Geometry check sheet. Reference: the model listing, model coordinates, mm. Face numbers are marked on the shaded views. A direction names the side the tool comes from. Round coordinates to 2 decimals unless told otherwise and drop trailing zeros. Loops run counter-clockwise (first coordinate to the right, second up) from the corner with the lowest first, then second, coordinate; pieces in that order, holes last. Notation, with made-up numbers: (37, 13.5) -> (43, 13.5) arc R32 ccw to (43, 50.5) -> close; hole circle Ø5 at (-2.75, -28). An arc over 180 degrees is marked (long way). Use a Markdown table: item, result. Add a question column.
Q1. Sectioned sample at A-A, the plane x = 8.75. Enter the section's corners in (y, z) (3 decimals).
Q2. Set-up check for the marked faces 1, 2, 3 and 4: record each of +Z, -Z, +X, -X, +Y, -Y from which the full face is reachable in a straight line by a thin tool's end or side.
Q3. Gauge pin test, flat ends, axial feed: P1, Ø2, axis at x = 1.5, z = 2.5, coming from the +Y side; P2, Ø5, axis at x = -5, y = 1, coming from the -Z side; P3, Ø4, axis at x = 4, z = -4.5, coming from the -Y side; P4, Ø3.5, axis at y = 1.5, z = -2, coming from the +X side (3 decimals). Record the tip position at first contact, or that the pin passes through.
Q4. Material ranges on L1, parallel to X at y = 4.25, z = 2; L2, parallel to X at y = 0, z = 5.5; L3, parallel to Z at x = -1, y = -3.75, recorded low to high.
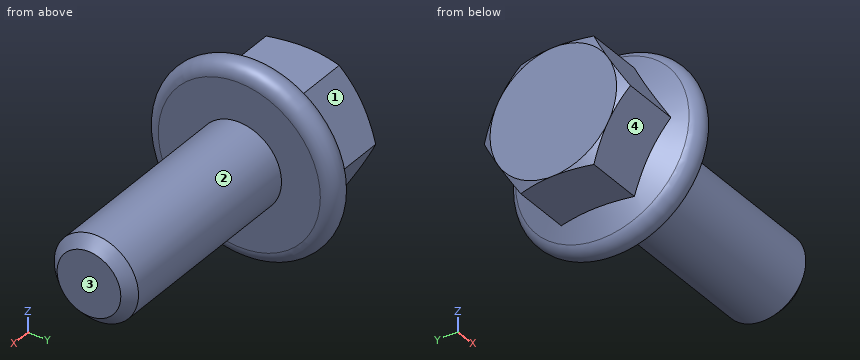
Autodesk Inventor part; units mm, degrees
ref_plane "Work Plane1" through (10.95, 0, 0) normal (0, 0, -1) x (1, 0, 0)
ref_plane "YZ Plane" through (0, 0, 0) normal (1, 0, 0) x (0, 1, 0)
ref_plane "XZ Plane" through (0, 0, 0) normal (0, 1, 0) x (-1, 0, 0)
sketch "Sketch1" plane through (0, 0, 0) normal (0, 0, 1) x (1, 0, 0)
  line L0 (-3.2004, 0) -> (-3.2004, 3.8156)
  line L1 (0, 6.096) -> (0, 3.175)
  line L2 (4.1148, 3.175) -> (15.875, 3.175)
  line L3 (15.875, 3.175) -> (15.875, 0)
  line L4 (15.875, 0) -> (-3.2004, 0)
  arc A0 (0, 6.096) -> (-1.9368, 6.5254) centre (-1.016, 6.096) ccw
  line L5 (0, -1.4605) -> (0, 8.7631)
  line L6 (-7.0155, 0) -> (19.6901, 0)
  line L7 (0, 3.175) -> (0.0001, 3.175)
  line L8 (0.0001, 3.175) -> (0.0001, 3.175)
  line L9 (0.0001, 3.175) -> (2.2098, 3.175)
  line L10 (2.2098, 3.175) -> (4.1148, 3.175)
  line L11 (-3.2004, 3.8156) -> (-1.9368, 6.5254)
  line L12 (0.0001, 3.175) -> (4.1148, 3.175) construction
  line L13 (4.1148, 3.175) -> (4.1148, 0) construction
  dimension "d0" = 1.016
  dimension "d1" = 15.875
  dimension "d2" = 11.7602
  dimension "d3" = 14.224
  dimension "d4" = 6.35
  dimension "d5" = 3.2004
  dimension "d15" = 6.35
  dimension "d16" = 6.35
  dimension "d17" = 0.0001
  dimension "d18" = 1.905
  dimension "d19" = 25
revolve "Body" add sketch "Sketch1" angle 360 about axis through (15.875, 0, 0) along (-1, 0, 0)
sketch "Sketch2" plane through (0, 0, 0) normal (1, 0, 0) x (0, 0, -1)
  line L0 (4.7625, 2.7496) -> (4.7625, -2.7496)
  line L1 (4.7625, -2.7496) -> (0, -5.4993)
  line L2 (0, -5.4993) -> (-4.7625, -2.7496)
  line L3 (-4.7625, -2.7496) -> (-4.7625, 2.7496)
  line L4 (-4.7625, 2.7496) -> (0, 5.4993)
  line L5 (0, 5.4993) -> (4.7625, 2.7496)
  point P0 (0, 0)
  point P1 (0, 0)
  dimension "d23" = 9.525
extrude "Head" add sketch "Sketch2" against normal blind 7.112
sketch "Sketch3" plane through (0, 0, 0) normal (0, 0, 1) x (1, 0, 0)
  line L0 (-7.112, 4.7625) -> (-7.112, 5.4993)
  line L1 (-7.112, 5.4993) -> (-6.6866, 5.4993)
  line L2 (-6.6866, 5.4993) -> (-7.112, 4.7625)
  line L3 (-8.0513, 0) -> (-1.476, 0)
  line L4 (-7.112, 5.4993) -> (-7.112, 2.7496)
  line L5 (-2.4153, 5.4993) -> (-7.112, 5.4993)
  point P0 (-7.112, 2.7496)
  dimension "d8" = 30
  dimension "d22" = 9.525
revolve "Chamfer1" cut sketch "Sketch3" angle 360 about axis through (-10, 0, 0) along (1, 0, 0)
thread "Thread"
chamfer "Chamfer2" distance 0.7791 distance2 0.7791 1 edges at (15.875, -3.175, 0) measured on face at (15.875, 0.0371, -1.7957)
ref_plane "Work Plane1" through (10.95, 0, 0) normal (0, 0, -1) x (1, 0, 0)
equation "\"d23\" = SW"
equation "\"d6\" = KOH"
equation "\"d10\" = GEL"
equation "\"d13\" = -0.5 * SPD + 0.5 * GD"
equation "\"d14\" = GUL"
equation "\"d0\" = PHH"
equation "\"d1\" = NLG"
equation "\"d2\" = GEL"
equation "\"d3\" = LADI"
equation "\"d4\" = GD"
equation "\"d5\" = 0.45 * KOH"
equation "\"d15\" = SD2"
equation "\"d16\" = BDM"
equation "\"d18\" = GAL"
equation "\"d19\" = KEWI"
equation "\"d8\" = ANG1"
equation "\"d22\" = SW0"
equation "\"NLG\" = 15.875"
equation "\"GD\" = NND"
equation "\"BDM\" = NND"
equation "\"KOH\" = 7.112"
equation "\"GEL\" = 11.7602"
equation "\"LADI\" = 14.224"
equation "\"SW\" = 9.525"
equation "\"PHH\" = 1.016"
equation "\"SW0\" = SW"
equation "\"SPD\" = 4.79184"
equation "\"SD2\" = NND"
equation "\"SD\" = 0"
equation "\"ANG1\" = 30deg"
equation "\"KEWI\" = 25deg"
equation "\"GAL\" = 1.905"
equation "\"GUL\" = 0.77908"
equation "\"THREADDIA\" = 6.35"
equation "\"SDH\" = SW"
equation "\"TOA\" = 30deg"
equation "\"NND\" = 6.35"
equation "\"E0\" = 1.155 * SW"
equation "\"GD1\" = 4.79184"
properties part number "92979A114" material "Steel, Mild"
Values:
| question | item | result |
|---|---|---|
| 1 | outline | circle Ø6.35 at (0, 0) |
| 2 | face 1 | +Z, -X, +Y |
| 2 | face 2 | +X |
| 2 | face 3 | +Z, -Z, +X, +Y, -Y |
| 2 | face 4 | -Z, -X, -Y |
| 3 | P1 | y = 2.8 |
| 3 | P2 | z = -5.24 |
| 3 | P3 | y = -1.96 |
| 3 | P4 | x = 15.875 |
| 4 | L1 | -7.11 to 0 |
| 4 | L2 | -2.41 to 0 |
| 4 | L3 | -6.04 to 6.04 |
